The listing builds one solid part. Answer for the finished solid, in the listing's coordinates (mm). Face numbers are marked on the shaded views. Give positions to 0.01 mm unless a question says otherwise; leave off trailing zeros.
```python
from build123d import *

# Parameters (mm, degrees)
BOSS_EXTRUDE2_DEPTH = 5
SKETCH7_R           = 1.5
CUT_EXTRUDE6_DEPTH  = 5
SKETCH2_R           = 1.5
CUT_EXTRUDE7_DEPTH  = 5
SKETCH4_R           = 1.5
CUT_EXTRUDE8_DEPTH  = 5
SKETCH10_R          = 1.5
CUT_EXTRUDE9_DEPTH  = 5
CUT_EXTRUDE10_DEPTH = 5
SKETCH15_R          = 1.5
CUT_EXTRUDE11_DEPTH = 161.15617378
CUT_EXTRUDE12_DEPTH = 5


with BuildPart() as part:
    # Sketch1 → Boss-Extrude2 (new body)
    with BuildSketch(Plane(origin=(0, 0, 0), x_dir=(1, 0, 0), z_dir=(0, 1, 0))):
        with BuildLine():
            Line((-120, 100), (-107.361996995, 100))
            Line((-107.361996995, 100), (-107.361996995, 80))
            Line((-107.361996995, 80), (-97.361996995, 70))
            Line((-97.361996995, 70), (-17.361996995, 70))
            Line((-17.361996995, 70), (-7.361996995, 80))
            Line((-7.361996995, 80), (-7.361996995, 100))
            Line((-7.361996995, 100), (1.39320225, 100))
            ThreePointArc((1.39320225, 100), (24.368494305, 97.324898947), (46.1145618, 89.4427191))
            Line((46.1145618, 89.4427191), (116.708203932, 54.145898034))
            ThreePointArc((116.708203932, 54.145898034), (122.759762125, 48.615456851), (125, 40.729490169))
            Line((125, 40.729490169), (125, -40.729490169))
            ThreePointArc((125, -40.729490169), (122.759762125, -48.615456851), (116.708203932, -54.145898034))
            Line((116.708203932, -54.145898034), (46.1145618, -89.4427191))
            ThreePointArc((46.1145618, -89.4427191), (24.368494305, -97.324898947), (1.39320225, -100))
            Line((1.39320225, -100), (-7.361996995, -100))
            Line((-7.361996995, -100), (-7.361996995, -80))
            Line((-7.361996995, -80), (-17.361996995, -70))
            Line((-17.361996995, -70), (-97.361996995, -70))
            Line((-97.361996995, -70), (-107.361996995, -80))
            Line((-107.361996995, -80), (-107.361996995, -100))
            Line((-107.361996995, -100), (-120, -100))
            ThreePointArc((-120, -100), (-123.535533906, -98.535533906), (-125, -95))
            Line((-125, -95), (-125, 95))
            ThreePointArc((-125, 95), (-123.535533906, 98.535533906), (-120, 100))
        make_face()
    extrude(amount=-BOSS_EXTRUDE2_DEPTH)

    # Sketch7 → Cut-Extrude6 (cut)
    with BuildSketch(Plane(origin=(0, 0, 0), x_dir=(1, 0, 0), z_dir=(0, 1, 0))):
        with Locations(Location((1.966861521, 27.998221343, 0), (0, 0, 270))):
            Circle(SKETCH7_R)
        with Locations(Location((71.966861521, 20.005897242, 0), (0, 0, 270))):
            Circle(SKETCH7_R)
        with Locations(Location((1.966861521, -28.001778657, 0), (0, 0, 270))):
            Circle(SKETCH7_R)
        with Locations(Location((71.966861521, -19.994102758, 0), (0, 0, 270))):
            Circle(SKETCH7_R)
        with BuildLine():
            Line((24.466861521, 10.195064991), (49.466861521, 10.195064991))
            ThreePointArc((49.466861521, 10.195064991), (51.234628473, 9.462831944), (51.966861521, 7.695064991))
            Line((51.966861521, 7.695064991), (51.966861521, -7.304935009))
            ThreePointArc((51.966861521, -7.304935009), (51.234628473, -9.072701962), (49.466861521, -9.804935009))
            Line((49.466861521, -9.804935009), (24.466861521, -9.804935009))
            ThreePointArc((24.466861521, -9.804935009), (22.699094568, -9.072701962), (21.966861521, -7.304935009))
            Line((21.966861521, -7.304935009), (21.966861521, 7.695064991))
            ThreePointArc((21.966861521, 7.695064991), (22.699094568, 9.462831944), (24.466861521, 10.195064991))
        make_face()
    extrude(amount=-CUT_EXTRUDE6_DEPTH, mode=Mode.SUBTRACT)

    # Sketch2 → Cut-Extrude7 (cut)
    with BuildSketch(Plane(origin=(0, 0, 0), x_dir=(1, 0, 0), z_dir=(0, 1, 0))):
        with Locations(Location((110, 17, 0), (0, 0, 270))):
            Circle(SKETCH2_R)
        with Locations(Location((110, -17, 0), (0, 0, 270))):
            Circle(SKETCH2_R)
    extrude(amount=-CUT_EXTRUDE7_DEPTH, mode=Mode.SUBTRACT)

    # Sketch4 → Cut-Extrude8 (cut)
    with BuildSketch(Plane(origin=(0, 0, 0), x_dir=(1, 0, 0), z_dir=(0, 1, 0))):
        with Locations(Location((-97.352664983, -24.5, 0), (0, 0, 270))):
            Circle(SKETCH4_R)
        with Locations(Location((-39.352664983, 24.5, 0), (0, 0, 270))):
            Circle(SKETCH4_R)
        with Locations(Location((-97.352664983, 24.5, 0), (0, 0, 270))):
            Circle(SKETCH4_R)
        with Locations(Location((-39.352664983, -24.5, 0), (0, 0, 270))):
            Circle(SKETCH4_R)
    extrude(amount=-CUT_EXTRUDE8_DEPTH, mode=Mode.SUBTRACT)

    # Sketch10 → Cut-Extrude9 (cut)
    with BuildSketch(Plane(origin=(0, 0, 0), x_dir=(1, 0, 0), z_dir=(0, 1, 0))):
        with Locations(Location((-100, 50.00070964, 0), (0, 0, 270))):
            Circle(SKETCH10_R)
        with Locations(Location((-100, -49.99929036, 0), (0, 0, 270))):
            Circle(SKETCH10_R)
        with Locations(Location((25, 75.00070964, 0), (0, 0, 270))):
            Circle(SKETCH10_R)
        with Locations(Location((25, -74.99929036, 0), (0, 0, 270))):
            Circle(SKETCH10_R)
    extrude(amount=-CUT_EXTRUDE9_DEPTH, mode=Mode.SUBTRACT)

    # Sketch11 → Cut-Extrude10 (cut)
    with BuildSketch(Plane(origin=(0, 0, 0), x_dir=(1, 0, 0), z_dir=(0, 1, 0))):
        with BuildLine():
            Line((43.618033989, 71.094545302), (90.527864045, 47.639630274))
            ThreePointArc((90.527864045, 47.639630274), (91.84295253, 44.829179995), (89.409830056, 42.903562297))
            Line((89.409830056, 42.903562297), (42.5, 42.903562297))
            ThreePointArc((42.5, 42.903562297), (40.732233047, 43.635795344), (40, 45.403562297))
            Line((40, 45.403562297), (40, 68.858477325))
            ThreePointArc((40, 68.858477325), (41.18567222, 70.985104346), (43.618033989, 71.094545302))
        make_face()
        with BuildLine():
            Line((40, -68.858477325), (40, -45.403562297))
            ThreePointArc((40, -45.403562297), (40.732233047, -43.635795344), (42.5, -42.903562297))
            Line((42.5, -42.903562297), (89.409830056, -42.903562297))
            ThreePointArc((89.409830056, -42.903562297), (91.84295253, -44.829179995), (90.527864045, -47.639630274))
            Line((90.527864045, -47.639630274), (43.618033989, -71.094545302))
            ThreePointArc((43.618033989, -71.094545302), (41.18567222, -70.985104346), (40, -68.858477325))
        make_face()
    extrude(amount=-CUT_EXTRUDE10_DEPTH, mode=Mode.SUBTRACT)

    # Sketch15 → Cut-Extrude11 (cut, through all)
    with BuildSketch(Plane(origin=(0, 0, 0), x_dir=(1, 0, 0), z_dir=(0, 1, 0))):
        with Locations(Location((92, 56.996711096, 0), (0, 0, 270))):
            Circle(SKETCH15_R)
        with Locations(Location((92, -56.996711096, 0), (0, 0, 90))):
            Circle(SKETCH15_R)
    extrude(amount=-CUT_EXTRUDE11_DEPTH, mode=Mode.SUBTRACT)

    # Sketch16 → Cut-Extrude12 (cut)
    with BuildSketch(Plane(origin=(0, 0, 0), x_dir=(1, 0, 0), z_dir=(0, 1, 0))):
        Polygon((-125, 28), (-120.6, 28), (-115, 22.4), (-115, -22.4), (-120.6, -28), (-125, -28), align=None)
    extrude(amount=-CUT_EXTRUDE12_DEPTH, mode=Mode.SUBTRACT)


solid = part.part
```
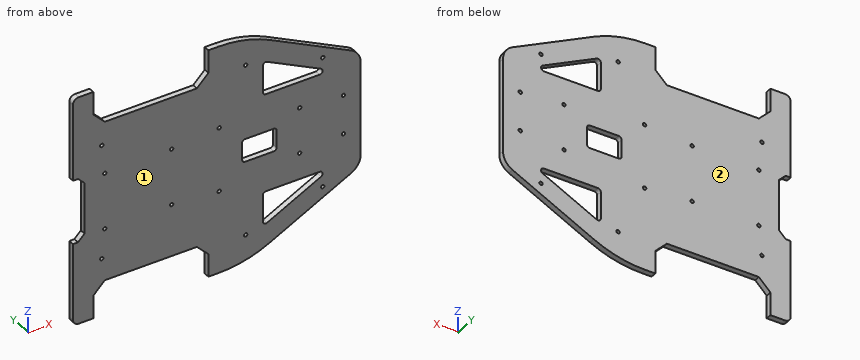
Item 1: A cutting plane is placed at A-A, the plane y = -1.7. Count the separate pieces of the cut face and the enclosed holes in it, plus the area to 3 significant figures.
Conclusion:
separate pieces: 1
enclosed holes: 19
area: 36,100 mm2
Item 2: Determine the mould class of the marked faces 1 and 2 for opening direction Y: pulls with the +Y half, pulls with the -Y half, needs draft (parallel to the pull), parting line crosses it, or undercut.
Conclusion:
face 1: pulls with the -Y half
face 2: pulls with the +Y half
Item 3: Each of these flat-tipped pins is pushed along its axis until it touches: P1, Ø1.5, axis at x = 35.5, y = -3, coming from the +Z side; P2, Ø2.5, axis at x = 40, y = -1.5, coming from the -Z side; P3, Ø1, axis at x = -90.5, y = -2.5, coming from the +Z side. Where does it stop, or does it pass through?
Conclusion:
P1: stops at z = 94.27
P2: stops at z = -92.76
P3: stops at z = 70
Item 4: Consider probe 1 along X at (y, z) = (-4.05, -23.5); probe 2 along Z at (x, y) = (-100.5, -1.65); probe 3 along X at (y, z) = (-1.75, 2.5). Determine where each line is inside the solid, lowest interval first.
Conclusion:
probe 1: x = -116.1 to -98.47, -96.23 to -40.47, -38.23 to 125
probe 2: z = -73.14 to -51.41, -48.59 to 48.59, 51.41 to 73.14
probe 3: x = -115 to 21.97, 51.97 to 125
